```python
from build123d import *

# Parameters (mm, degrees)
SKETCH_1_R          = 5
SKETCH_1_R_2        = 1.55
EXTRUDE_1_DEPTH     = 4.75
SKETCH_2_R          = 2.75
SKETCH_2_R_2        = 1.55
EXTRUDE_2_DEPTH     = 2
SKETCH_3_R          = 3.5
SKETCH_3_R_2        = 1.55
CUT_EXTRUDE_1_DEPTH = 2


with BuildPart() as part:
    # 草图1 → 凸台-拉伸1 (new body)
    with BuildSketch(Plane.XY):
        Circle(SKETCH_1_R)
        Circle(SKETCH_1_R_2, mode=Mode.SUBTRACT)
    extrude(amount=EXTRUDE_1_DEPTH)

    # 草图2 → 凸台-拉伸2 (add)
    with BuildSketch(Plane.XY.offset(4.75)):
        Circle(SKETCH_2_R)
        Circle(SKETCH_2_R_2, mode=Mode.SUBTRACT)
    extrude(amount=EXTRUDE_2_DEPTH)

    # 草图3 → 切除-拉伸1 (cut)
    with BuildSketch(Plane(origin=(0, 0, 0), x_dir=(-1, 0, 0), z_dir=(0, 0, -1))):
        Circle(SKETCH_3_R)
        Circle(SKETCH_3_R_2, mode=Mode.SUBTRACT)
    extrude(amount=-CUT_EXTRUDE_1_DEPTH, mode=Mode.SUBTRACT)


solid = part.part
```
Geometry: final body of the model. Coordinates: model frame, mm. A direction names the side the tool comes from. Give positions to 0.01 mm unless a question says otherwise; leave off trailing zeros. Loops run counter-clockwise (first coordinate to the right, second up) from the corner with the lowest first, then second, coordinate; pieces in that order, holes last. Notation, with made-up numbers: (36, 66.25) -> (42, 66.25) arc R31 cw to (42, 90.25) -> close; hole circle Ø9 at (-26.5, 89.5). An arc over 180 degrees is marked (long way). Return JSON: item names as keys, results as strings.
Item 1: Access query for faces 4 (the flat face through (-1, -2, 2)), 5 (the flat face through (2.2, -2.2, 4.75)), 6 (the flat face through (2.2, -3.3, 0)). Directions: +Z, -Z, +X, -X, +Y, -Y. A direction counts if a zero-diameter tool reaches every point of the face in a straight line with its end or side. Return the directions, or none.
Filled in:
{"face 4": "-Z", "face 5": "+Z", "face 6": "-Z, +X, -X, +Y, -Y"}
Item 2: Section A-A, the plane y = 0. Output: boundary loops of the cut face in (x, z), plus the area to 3 significant figures.
Filled in:
{"outline": "(-5, 0) -> (-3.5, 0) -> (-3.5, 2) -> (-1.55, 2) -> (-1.55, 6.75) -> (-2.75, 6.75) -> (-2.75, 4.75) -> (-5, 4.75) -> close; (1.55, 2) -> (3.5, 2) -> (3.5, 0) -> (5, 0) -> (5, 4.75) -> (2.75, 4.75) -> (2.75, 6.75) -> (1.55, 6.75) -> close", "area": "29.8 mm^2"}
Item 3: Section D-D, the plane x = 1.75. Output: boundary loops of the cut face in (y, z).
Filled in:
{"outline": "(-4.68, 0) -> (-3.03, 0) -> (-3.03, 2) -> (3.03, 2) -> (3.03, 0) -> (4.68, 0) -> (4.68, 4.75) -> (2.12, 4.75) -> (2.12, 6.75) -> (-2.12, 6.75) -> (-2.12, 4.75) -> (-4.68, 4.75) -> close"}
Item 4: Pin query (flat end, axial travel): P1, Ø2, axis at x = -4, z = 2, coming from the -Y side; P2, Ø1.9, axis at x = 0, y = 0, coming from the +Z side; P3, Ø1.5, axis at y = 2.5, z = 5, coming from the -X side. Return the tip coordinate at first contact, or that it passes through.
Filled in:
{"P1": "y = -4", "P2": "through", "P3": "x = -4.67"}
Item 5: Line query: line 1 (Y direction, x = 0, z = 1.4); line 2 (Y direction, x = 0, z = 3.75); line 3 (Z direction, x = -1.5, y = 2.5). Output: solid intervals per line, ascending.
Filled in:
{"line 1": "-5 to -3.5, 3.5 to 5", "line 2": "-5 to -1.55, 1.55 to 5", "line 3": "2 to 4.75"}
Item 6: Section C-C, the plane z = 4.5. Output: boundary loops of the cut face in (x, y), plus the area to 3 significant figures.
Filled in:
{"outline": "circle Ø10 at (0, 0); hole circle Ø3.1 at (0, 0)", "area": "71.0 mm^2"}
Item 7: Mould query, pull axis Y, two halves, no side actions, for faces 1 (the cylindrical face through (-0.596, -2.685, 5.736)), 2 (the cylindrical face through (-3.233, -1.341, 0.986)), 3 (the flat face through (2, 0, 6.75)). Classes: released by +Y, released by -Y, zero draft, split by the parting line, or undercut.
Filled in:
{"face 1": "split by the parting line", "face 2": "undercut", "face 3": "zero draft"}
